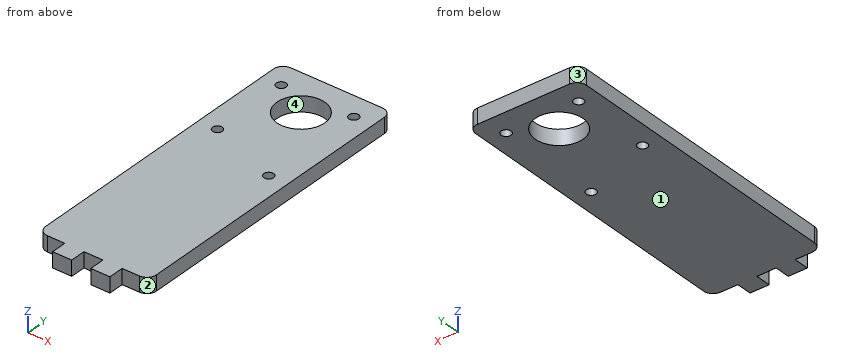
from build123d import *

# Parameters (mm, degrees)
SKETCH1_W           = 58
SKETCH1_H           = 160
BOSS_EXTRUDE1_DEPTH = 8
SKETCH2_R           = 2.55
SKETCH2_R_2         = 12.5
CUT_EXTRUDE1_DEPTH  = 86.469292731
SKETCH6_W           = 10
SKETCH6_H           = 8
BOSS_EXTRUDE3_DEPTH = 8
FILLET2_R           = 5


with BuildPart() as part:
    # Sketch1 → Boss-Extrude1 (new body)
    with BuildSketch(Plane.XY):
        Rectangle(SKETCH1_W, SKETCH1_H)
    extrude(amount=BOSS_EXTRUDE1_DEPTH)

    # Sketch2 → Cut-Extrude1 (cut, through all)
    with BuildSketch(Plane.XY.offset(8)):
        with Locations((-19, 67.5)):
            Circle(SKETCH2_R)
        with Locations((19, 67.5)):
            Circle(SKETCH2_R)
        with Locations((-19, 25.5)):
            Circle(SKETCH2_R)
        with Locations((19, 11.5)):
            Circle(SKETCH2_R)
        with Locations((0, 56.5)):
            Circle(SKETCH2_R_2)
    extrude(amount=-CUT_EXTRUDE1_DEPTH, mode=Mode.SUBTRACT)

    # Sketch6 → Boss-Extrude3 (add)
    with BuildSketch(Plane.XZ.offset(80)):
        with Locations((-10, 4)):
            Rectangle(SKETCH6_W, SKETCH6_H)
        with Locations((10, 4)):
            Rectangle(SKETCH6_W, SKETCH6_H)
    extrude(amount=BOSS_EXTRUDE3_DEPTH)

    # Fillet2
    fillet2_edges = [part.edges().sort_by_distance(p)[0] for p in [
        (29, 80, 4),
        (-29, 80, 4),
        (29, -80, 4),
        (-29, -80, 4),
    ]]
    fillet(fillet2_edges, radius=FILLET2_R)


solid = part.part
The listing builds one solid part. Answer for the finished solid, in the listing's coordinates (mm). Face numbers are marked on the shaded views. Give positions to 0.01 mm unless a question says otherwise; leave off trailing zeros. Loops run counter-clockwise (first coordinate to the right, second up) from the corner with the lowest first, then second, coordinate; pieces in that order, holes last.
Item 1: Each of these flat-tipped pins is pushed along its axis until it touches: pin 1 Ø4.5 at (x, y) = (19, 11.5) entering from +Z; pin 2 Ø1 at (x, z) = (21, 1.5) entering from -Y; pin 3 Ø4 at (x, y) = (16.5, -32) entering from -Z; pin 4 Ø2.5 at (y, z) = (-84, 5) entering from -X. Where does it stop, or does it pass through?
Derived:
pin 1: passes through
pin 2: stops at y = -80
pin 3: stops at z = 0
pin 4: stops at x = -15
Item 2: A cutting plane is placed at B-B (z = 4). Give the vertices of the cut face in (x, y).
Derived:
outline: (-29, -75) arc R5 ccw to (-24, -80) - (-15, -80) - (-15, -88) - (-5, -88) - (-5, -80) - (5, -80) - (5, -88) - (15, -88) - (15, -80) - (24, -80) arc R5 ccw to (29, -75) - (29, 75) arc R5 ccw to (24, 80) - (-24, 80) arc R5 ccw to (-29, 75) - close; hole circle Ø5.1 at (-19, 25.5); hole circle Ø5.1 at (-19, 67.5); hole circle Ø25 at (0, 56.5); hole circle Ø5.1 at (19, 11.5); hole circle Ø5.1 at (19, 67.5)
Item 3: A cutting plane is placed at D-D (y = 56.5). Give the vertices of the cut face in (x, z).
Derived:
outline: (-29, 0) - (-12.5, 0) - (-12.5, 8) - (-29, 8) - close; (12.5, 0) - (29, 0) - (29, 8) - (12.5, 8) - close
Item 4: Determine the mould class of the marked faces 1, 2, 3 and 4 for opening direction Y: +Y half, -Y half, draft (parallel to the pull), parting line (faces both ways), or undercut.
Derived:
face 1: draft
face 2: -Y half
face 3: +Y half
face 4: undercut
Item 5: A cutting plane is placed at C-C (x = -19). Give the vertices of the cut face in (y, z), then the cut area to 3 significant figures.
Derived:
outline: (-80, 0) - (22.95, 0) - (22.95, 8) - (-80, 8) - close; (28.05, 0) - (64.95, 0) - (64.95, 8) - (28.05, 8) - close; (70.05, 0) - (80, 0) - (80, 8) - (70.05, 8) - close
area: 1,200 mm2
Item 6: A cutting plane is placed at A-A (x = -7.5). Give the vertices of the cut face in (y, z), then the cut area to 3 significant figures.
Derived:
outline: (-88, 0) - (46.5, 0) - (46.5, 8) - (-88, 8) - close; (66.5, 0) - (80, 0) - (80, 8) - (66.5, 8) - close
area: 1,180 mm2
Item 7: Find the intervals of material crossed by line 1 along Y through (x, z) = (-19, 4.5); line 2 along Y through (x, z) = (19, 4.5); line 3 along X through (y, z) = (66.5, 1), in increasing order.
Derived:
line 1: y = -80 to 22.95, 28.05 to 64.95, 70.05 to 80
line 2: y = -80 to 8.95, 14.05 to 64.95, 70.05 to 80
line 3: x = -29 to -21.35, -16.65 to -7.5, 7.5 to 16.65, 21.35 to 29
